Part model, mm, in its own coordinate system. Face numbers are marked on the shaded views. A direction names the side the tool comes from. Give positions to 0.01 mm unless a question says otherwise; leave off trailing zeros. Write each loop counter-clockwise with the first axis right and the second up, starting at its lowest first coordinate (ties: lowest second). Pieces come first, ordered by that corner, then holes.
Autodesk Inventor part; units mm, degrees
ref_plane "YZ Plane" through (0, 0, 0) normal (1, 0, 0) x (0, 1, 0)
ref_plane "XZ Plane" through (0, 0, 0) normal (0, 1, 0) x (-1, 0, 0)
ref_plane "XY Plane" through (0, 0, 0) normal (0, 0, 1) x (1, 0, 0)
sketch "Szkic1" plane through (0, 0, 0) normal (0, 0, 1) x (1, 0, 0)
  circle A0 centre (0, 0) radius 2.5
  circle A1 centre (0, 0) radius 9.5
  dimension "d0" = 5
  dimension "d1" = 19
extrude "Wyciągnięcie proste1" add sketch "Szkic1" along normal blind 6
chamfer "Faza1" distance 0.3 angle 45 4 edges at (-9.5, 0, 6) (-2.5, 0, 6) (-9.5, 0, 0) (-2.5, 0, 0)
sketch "Szkic2" plane through (0, 0, 0) normal (0, 0, -1) x (-1, 0, 0)
  circle A0 centre (0, 0) radius 9.2
  circle A1 centre (0, 0) radius 2.8
  circle A2 centre (0, 0) radius 9.5
  circle A3 centre (0, 0) radius 2.5
  circle A4 centre (0, 0) radius 4.5
  circle A5 centre (0, 0) radius 8.5
  dimension "d7" = 2
  dimension "d8" = 1
extrude "Wyciągnięcie proste2" cut sketch "Szkic2" against normal blind 0.5 contours A5
sketch "Szkic3" plane through (0, 0, 6) normal (0, 0, 1) x (1, 0, 0)
  circle A0 centre (0, 0) radius 8.5
  circle A1 centre (0, 0) radius 4.5
extrude "Wyciągnięcie proste3" cut sketch "Szkic3" against normal blind 0.5
properties part number "COTS_GENERIC_Bearing_19x5x6"
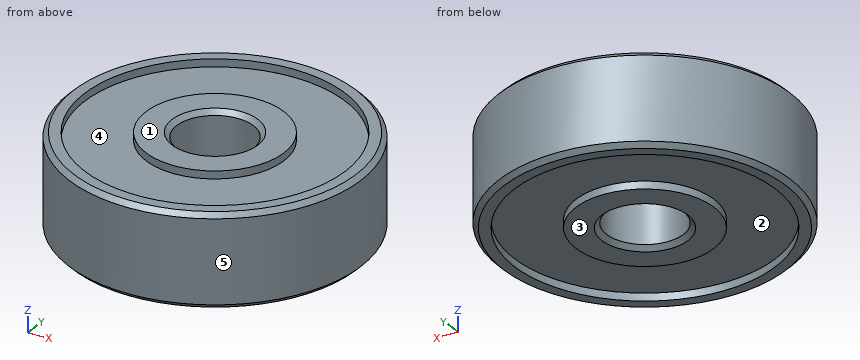
1) 3-axis set-ups, long thin cutter, end or side, ignore diameter. For the marked faces 1 and 2: which of +Z, -Z, +X, -X, +Y, -Y reach the whole face in a straight line?
Answers follow:
face 1: +Z, +X, -X, +Y, -Y
face 2: -Z
2) Saw through at B-B, the plane z = 1.55. Write the cut outline in (x, y).
Answers follow:
outline: circle Ø19 at (0, 0); hole circle Ø5 at (0, 0)
3) Two-plate mould, pull along Y, no slides. Class the marked faces 3, 4 and 5: +Y half, -Y half, draft (parallel to the pull), parting line (faces both ways), or undercut.
Answers follow:
face 3: draft
face 4: undercut
face 5: parting line
4) Pin check, flat tips, straight feed: pin 1 Ø2 at (x, y) = (-6, 5) entering from +Z; pin 2 Ø1.5 at (x, z) = (-6, 5) entering from -Y; pin 3 Ø1 at (x, z) = (-6, 1.5) entering from -Y; pin 4 Ø3 at (x, z) = (-4.5, 4.5) entering from +Y. Stop position of each tip, or through.
Answers follow:
pin 1: stops at z = 6
pin 2: stops at y = -7.92
pin 3: stops at y = -7.75
pin 4: stops at y = 9.01
5) Wall check: L1, parallel to Z at x = -3, y = 5.5; L2, parallel to Y at x = -1, z = 3.6; L3, parallel to Y at x = 0.5, z = 5.1. Give the ranges that are in metal, low to high.
Answers follow:
L1: z = 0.5 to 5.5
L2: y = -9.45 to -2.29, 2.29 to 9.45
L3: y = -9.49 to -2.45, 2.45 to 9.49
